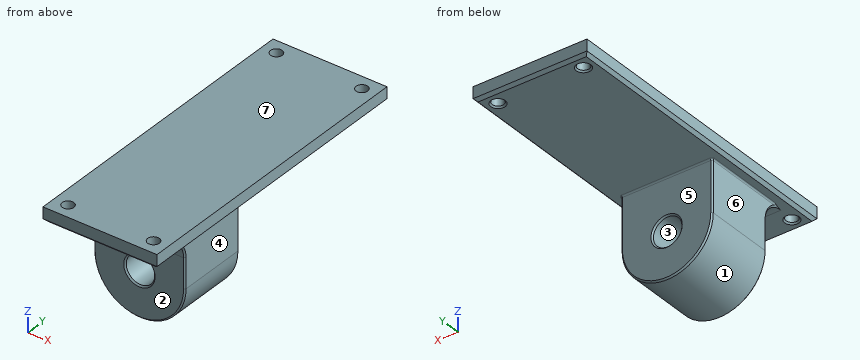
```python
from build123d import *

# Parameters (mm, degrees)
SKETCH1_W                  = 80
SKETCH1_H                  = 213
BOSS_EXTRUDE1_DEPTH        = 10
BOSS_EXTRUDE2_START        = -20
BOSS_EXTRUDE2_DEPTH        = 50
FILLET1_R                  = 15
SKETCH3_R                  = 10
CUT_EXTRUDE1_DEPTH         = 150.084707465
CHAMFER1_SIZE              = 1
F_8_2_8_2_DIAMETER_HOLE1_D = 8.2
CHAMFER2_SIZE              = 2
CHAMFER3_SIZE              = 1
FILLET2_R                  = 1


with BuildPart() as part:
    # Sketch1 → Boss-Extrude1 (new body)
    with BuildSketch(Plane.XY):
        Rectangle(SKETCH1_W, SKETCH1_H)
    extrude(amount=BOSS_EXTRUDE1_DEPTH)

    # Sketch2 → Boss-Extrude2 (add)
    with BuildSketch(Plane(origin=(0, 0, 0), x_dir=(1, 0, 0), z_dir=(0, 1, 0)).offset(BOSS_EXTRUDE2_START)):
        with BuildLine():
            Line((-32, 36), (-32, 0))
            Line((-32, 0), (32, 0))
            Line((32, 0), (32, 36))
            ThreePointArc((32, 36), (0, 68), (-32, 36))
        make_face()
    extrude(amount=-BOSS_EXTRUDE2_DEPTH)

    # Fillet1
    fillet1_edges = [part.edges().sort_by_distance(p)[0] for p in [
        (0, -70, 0),
    ]]
    fillet(fillet1_edges, radius=FILLET1_R)

    # Sketch3 → Cut-Extrude1 (cut, through all)
    with BuildSketch(Plane(origin=(0, -20, 0), x_dir=(1, 0, 0), z_dir=(0, 1, 0))):
        with Locations(Location((0, 36, 0), (0, 0, 270))):
            Circle(SKETCH3_R)
    extrude(amount=-CUT_EXTRUDE1_DEPTH, mode=Mode.SUBTRACT)

    # Chamfer1
    # the kernel refuses this chamfer: 1 mm, written as the material it takes off along each edge
    with BuildSketch(Plane(origin=(0, -70, -36), x_dir=(1, 0, 0), z_dir=(0, 0, 1))) as chamfer1_piece_1:
        Polygon((32 - CHAMFER1_SIZE, 0), (32, CHAMFER1_SIZE), (32, 0), align=None)
    revolve(axis=Axis((0, -70, -36), (0, 1, 0)), revolution_arc=180, mode=Mode.SUBTRACT)
    with BuildSketch(Plane(origin=(-32, -70, -36), x_dir=(-0.027495876610589196, 0.9996219169112968, 0), z_dir=(0, 0, 1)), Plane(origin=(32, -70, -15), x_dir=(0.027495876610589196, 0.9996219169112968, 0), z_dir=(0, 0, -1))) as chamfer1_piece_2:
        Polygon((CHAMFER1_SIZE * 0.999621916911, -CHAMFER1_SIZE * 0.0274958766106), (-CHAMFER1_SIZE * 0.0274958766106, -CHAMFER1_SIZE * 0.999621916911), (0, 0), align=None)
    extrude(amount=21, mode=Mode.SUBTRACT)
    with BuildSketch(Plane(origin=(0, -20, -36), x_dir=(1, 0, 0), z_dir=(0, 0, 1))) as chamfer1_piece_3:
        Polygon((32 - CHAMFER1_SIZE, 0), (32, -CHAMFER1_SIZE), (32, 0), align=None)
    revolve(axis=Axis((0, -20, -36), (0, 1, 0)), revolution_arc=180, mode=Mode.SUBTRACT)
    with BuildSketch(Plane(origin=(-32, -20, -36), x_dir=(-0.0274958766105891, -0.9996219169112968, 0), z_dir=(0, 0, 1)), Plane(origin=(32, -20, 0), x_dir=(0.0274958766105891, -0.9996219169112968, 0), z_dir=(0, 0, -1))) as chamfer1_piece_4:
        Polygon((CHAMFER1_SIZE * 0.999621916911, CHAMFER1_SIZE * 0.0274958766106), (-CHAMFER1_SIZE * 0.0274958766106, CHAMFER1_SIZE * 0.999621916911), (0, 0), align=None)
    extrude(amount=36, mode=Mode.SUBTRACT)
    with BuildSketch(Plane(origin=(32, -85, -15), x_dir=(0, -0.17067472761230248, 0.9853274264702401), z_dir=(0, -0.9853274264702401, -0.17067472761230248))) as chamfer1_piece_5_section:
        Polygon((15, CHAMFER1_SIZE), (15 + CHAMFER1_SIZE, 0), (15, 0), align=None)
    chamfer1_piece_5 = revolve(axis=Axis((32, -85, -15), (-1, 0, 0)), revolution_arc=99.827051452, mode=Mode.PRIVATE)
    chamfer1_piece_5 = split(chamfer1_piece_5, bisect_by=Plane(origin=(31.514748262, -74.050273487, 0), z_dir=(0, 0, -1)), keep=Keep.TOP, mode=Mode.PRIVATE)
    add(chamfer1_piece_5, mode=Mode.SUBTRACT)
    with BuildSketch(Plane(origin=(-32, -85, -15), x_dir=(0, -0.17067472761230248, 0.9853274264702401), z_dir=(0, -0.9853274264702401, -0.17067472761230248))) as chamfer1_piece_6_section:
        Polygon((15 + CHAMFER1_SIZE, 0), (15, -CHAMFER1_SIZE), (15, 0), align=None)
    chamfer1_piece_6 = revolve(axis=Axis((-32, -85, -15), (-1, 0, 0)), revolution_arc=99.827051452, mode=Mode.PRIVATE)
    chamfer1_piece_6 = split(chamfer1_piece_6, bisect_by=Plane(origin=(-31.514748262, -74.050273487, 0), z_dir=(0, 0, -1)), keep=Keep.TOP, mode=Mode.PRIVATE)
    add(chamfer1_piece_6, mode=Mode.SUBTRACT)

    # Ø8.2 (8.2) Diameter Hole1 (through all)
    with Locations(Plane(origin=(0, 0, 0), x_dir=(-1, 0, 0), z_dir=(0, 0, -1))):
        with Locations((30, -96.5), (-30, 96.5), (-30, -96.5), (30, 96.5)):
            Hole(F_8_2_8_2_DIAMETER_HOLE1_D / 2)

    # Chamfer2
    chamfer2_edges = [part.edges().sort_by_distance(p)[0] for p in [
        (0, 106.5, 0),
        (40, 0, 0),
        (0, -106.5, 0),
        (-40, 0, 0),
    ]]
    chamfer(chamfer2_edges, length=CHAMFER2_SIZE)

    # Chamfer3
    chamfer3_edges = [part.edges().sort_by_distance(p)[0] for p in [
        (25.9, -96.5, 0),
        (25.9, 96.5, 0),
        (-34.1, -96.5, 0),
        (0, -70, -46),
        (0, -20, -46),
        (-34.1, 96.5, 0),
    ]]
    chamfer(chamfer3_edges, length=CHAMFER3_SIZE)

    # Fillet2
    fillet2_edges = [part.edges().sort_by_distance(p)[0] for p in [
        (-32, -50.216117819, 0),
        (32, -50.216117819, 0),
        (0, -20, 0),
        (-31.5, -20.5, 0),
        (31.5, -20.5, 0),
    ]]
    fillet(fillet2_edges, radius=FILLET2_R)


solid = part.part
```
Could you check a few things on this model? Use its own coordinates, in mm. Face numbers are marked on the shaded views. A direction names the side the tool comes from. Give positions to 0.01 mm unless a question says otherwise; leave off trailing zeros. Loops run counter-clockwise (first coordinate to the right, second up) from the corner with the lowest first, then second, coordinate; pieces in that order, holes last. Notation, with made-up numbers: (49.25, 89.5) -> (62.25, 89.5) arc R32 ccw to (62.25, 121.5) -> close; hole circle Ø2 at (86, -15.5). An arc over 180 degrees is marked (long way). Put each result on its own line as item: value.
(1) Imagine slicing it at C-C on y = -49. Write out the boundary of the cut face in (x, z), plus the area to 3 significant figures.
Computed:
outline: (-40, 2) -> (-38, 0) -> (-33, 0) arc R1 cw to (-32, -1) -> (-32, -36) arc R32 ccw to (32, -36) -> (32, -1) arc R1 cw to (33, 0) -> (38, 0) -> (40, 2) -> (40, 10) -> (-40, 10) -> close; hole circle Ø20 at (0, -36)
area: 4,390 mm^2
(2) Please list where these lines run through material, in increasing order: probe 1 along Y at (x, z) = (-30, 5); probe 2 along X at (y, z) = (-96, 5); probe 3 along X at (y, z) = (-52, -36). Write a range as [from, to].
Computed:
probe 1: [-106.5, -100.6], [-92.4, 92.4], [100.6, 106.5]
probe 2: [-40, -34.07], [-25.93, 25.93], [34.07, 40]
probe 3: [-32, -10], [10, 32]
(3) Imagine slicing it at D-D on y = -5. Write out the boundary of the cut face in (x, z), plus the area to 3 significant figures.
Computed:
outline: (-40, 2) -> (-38, 0) -> (38, 0) -> (40, 2) -> (40, 10) -> (-40, 10) -> close
area: 796 mm^2
(4) For the marked faces 4, 5, 6 and 7, which set-ups out of +Z, -Z, +X, -X, +Y, -Y let a thin tool reach every point of the face, with its end or its side?
Computed:
face 4: -Z, +X, +Y, -Y
face 5: -Z, +X, -X, +Y
face 6: -Z, -X, +Y, -Y
face 7: +Z, +X, -X, +Y, -Y
(5) I'm going to push flat-ended pins straight in: pin 1 Ø10.5 at (y, z) = (-54, -14) entering from -X; pin 2 Ø1.5 at (x, y) = (28.5, 74.5) entering from -Z; pin 3 Ø4 at (x, z) = (-17.5, -13) entering from -Y; pin 4 Ø13 at (x, y) = (-30, -96.5) entering from +Z. Where does each tip first touch, or does it pass through?
Computed:
pin 1: x = -32
pin 2: z = 0
pin 3: y = -70.54
pin 4: z = 10
(6) Imagine slicing it at B-B on y = -96.5. Write out the boundary of the cut face in (x, z), plus the area to 3 significant figures.
Computed:
outline: (-40, 2) -> (-38, 0) -> (-35.1, 0) -> (-34.1, 1) -> (-34.1, 10) -> (-40, 10) -> close; (-25.9, 1) -> (-24.9, 0) -> (24.9, 0) -> (25.9, 1) -> (25.9, 10) -> (-25.9, 10) -> close; (34.1, 1) -> (35.1, 0) -> (38, 0) -> (40, 2) -> (40, 10) -> (34.1, 10) -> close
area: 630 mm^2
(7) Imagine slicing it at A-A on x = 0. Write out the boundary of the cut face in (y, z), plus the area to 3 significant figures.
Computed:
outline: (-106.5, 2) -> (-104.5, 0) -> (-85, 0) arc R15 cw to (-70, -15) -> (-70, -25) -> (-69, -26) -> (-21, -26) -> (-20, -25) -> (-20, -1) arc R1 cw to (-19, 0) -> (104.5, 0) -> (106.5, 2) -> (106.5, 10) -> (-106.5, 10) -> close; (-70, -67) -> (-69, -68) -> (-21, -68) -> (-20, -67) -> (-20, -47) -> (-21, -46) -> (-69, -46) -> (-70, -47) -> close
area: 4,570 mm^2
(8) Thinking about a two-plate mould opening in X: for the marked faces 1, 2 and 3, which applies, pulls with the +X half, pulls with the -X half, needs draft (parallel to the pull), parting line crosses it, or undercut?
Computed:
face 1: parting line crosses it
face 2: needs draft
face 3: undercut
